The figure shows three views and two pictorial views of one solid part (mm, origin at its lowest corner). Answer the questions. A direction names the side the tool comes from. Round coordinates to 2 decimals unless told otherwise and drop trailing zeros. Order: outer loops, then holes, each group sorted by start corner. A loop starts at its lowest first (then second) coordinate and runs counter-clockwise, first axis right, second up. Notation, with made-up numbers: (81.25, 75.5) - (130.25, 75.5) arc R16 ccw to (130.25, 87.5) - close; hole circle Ø8 at (28.5, 56.25). An arc over 180 degrees is marked (long way). One line per item, written item: value. Start each with the question number.
1. Flat-ended cylindrical pins translate along their axes: P1, Ø4.5, axis at x = 20.75, z = 9.5, coming from the -Y side; P2, Ø9, axis at x = 34.5, z = 7, coming from the -Y side; P3, Ø5.5, axis at x = 23.5, y = 1.5, coming from the -Z side; P4, Ø4, axis at y = 1.5, z = 19, coming from the +X side. Find the tip coordinate at first contact, or state that the pin passes through.
2. Section B-B, the plane x = 7 is taken. Give the vertices of the cut face in (y, z), then the cut area to 3 significant figures.
3. Section A-A, the plane z = 33 is taken. Give the vertices of the cut face in (x, y), then the cut area to 4 significant figures.
4. For a pull along Z with two mould halves and no side action, classify the marked faces 4, 5, 6 and 7 as released by +Z, released by -Z, zero draft, split by the parting line, or undercut.
5. Section D-D, the plane z = 8.5 is taken. Give the vertices of the cut face in (x, y).
6. A tool of negligible diameter and unlimited length cuts with its end or side. For the marked faces 1, 2 and 3, from which of +Z, -Z, +X, -X, +Y, -Y can it reach the whole face along a straight path? Write none if from no direction.
7. Section C-C, the plane y = 13.5 is taken. Give the vertices of the cut face in (x, z).
8. Straight lines are drawn through the part: line 1 (Z direction, x = 34.5, y = 14.75); line 2 (Z direction, x = 20.75, y = 14); line 3 (Y direction, x = 31.5, z = 22). For each, find the intervals that lie inside material, in ascending order.
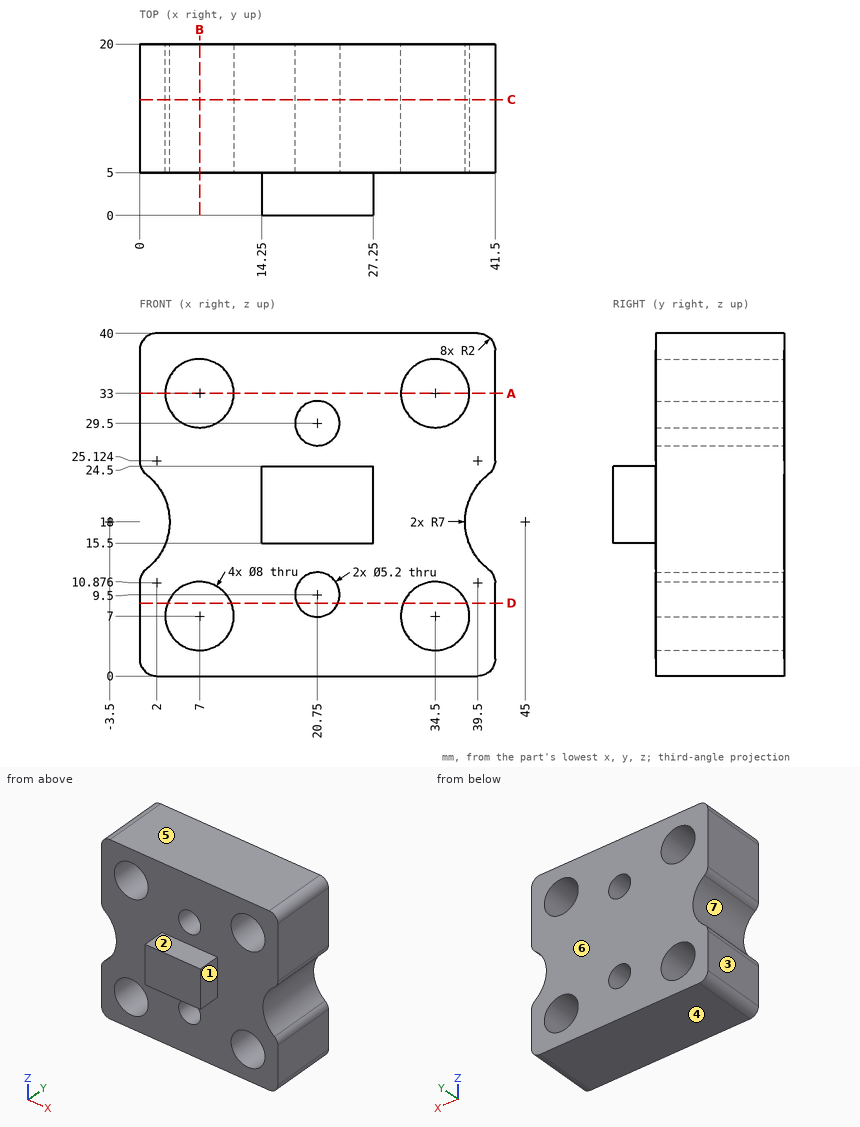
Answer list:
1. P1: passes through
1. P2: stops at y = 5
1. P3: stops at z = 15.5
1. P4: stops at x = 27.25
2. outline: (5, 0) - (20, 0) - (20, 3) - (5, 3) - close; (5, 11) - (20, 11) - (20, 29) - (5, 29) - close; (5, 37) - (20, 37) - (20, 40) - (5, 40) - close
2. area: 360 mm²
3. outline: (0, 5) - (3, 5) - (3, 20) - (0, 20) - close; (11, 5) - (30.5, 5) - (30.5, 20) - (11, 20) - close; (38.5, 5) - (41.5, 5) - (41.5, 20) - (38.5, 20) - close
3. area: 382.5 mm²
4. face 4: released by -Z
4. face 5: released by +Z
4. face 6: zero draft
4. face 7: undercut
5. outline: (0, 5) - (3.29, 5) - (3.29, 20) - (0, 20) - close; (10.71, 5) - (18.35, 5) - (18.35, 20) - (10.71, 20) - close; (23.15, 5) - (30.79, 5) - (30.79, 20) - (23.15, 20) - close; (38.21, 5) - (41.5, 5) - (41.5, 20) - (38.21, 20) - close
6. face 1: +Z, -Z, +X, -Y
6. face 2: +Z, +X, -X, -Y
6. face 3: +Z, -Z, -X, +Y, -Y
7. outline: (0, 2) arc R2 ccw to (2, 0) - (39.5, 0) arc R2 ccw to (41.5, 2) - (41.5, 10.88) arc R2 ccw to (40.72, 12.46) arc R7 cw to (40.72, 23.54) arc R2 ccw to (41.5, 25.12) - (41.5, 38) arc R2 ccw to (39.5, 40) - (2, 40) arc R2 ccw to (0, 38) - (0, 25.12) arc R2 ccw to (0.78, 23.54) arc R7 cw to (0.78, 12.46) arc R2 ccw to (0, 10.88) - close; hole circle Ø8 at (7, 7); hole circle Ø8 at (7, 33); hole circle Ø5.2 at (20.75, 9.5); hole circle Ø5.2 at (20.75, 29.5); hole circle Ø8 at (34.5, 7); hole circle Ø8 at (34.5, 33)
8. line 1: z = 0 to 3, 11 to 29, 37 to 40
8. line 2: z = 0 to 6.9, 12.1 to 26.9, 32.1 to 40
8. line 3: y = 5 to 20
